Geometry: final body of the model. Coordinates: model frame, mm. A direction names the side the tool comes from. Coordinates: 2 decimals unless noted, no trailing zeros. Write each loop counter-clockwise with the first axis right and the second up, starting at its lowest first coordinate (ties: lowest second). Pieces come first, ordered by that corner, then holes. Notation, with made-up numbers: M 32.5,43 L 63.5,43 A22 cw 63.5,62 Z; hole C 3.5,-10.5 d5. An arc over 180 degrees is marked long. Write item = value, one per line. Start each with the question number.
Item 1: First-contact query: pin 1 Ø5.5 at (y, z) = (28.5, 5.5) entering from +X; pin 2 Ø22.5 at (x, y) = (0, 0) entering from -Z; pin 3 Ø6 at (y, z) = (-35.5, 10) entering from -X; pin 4 Ø8 at (x, z) = (56.5, 16) entering from +Y. Flat tips, straight axial feed; report the tip coordinate or a pass-through.
Item 2: Pull-direction query (Y, two-part tool) for faces 5 (the cylindrical face through (107.144, 43.072, 9.392)), 6 (the cylindrical face through (-107.144, -43.072, 9.392)), 7 (the cylindrical face through (-2.447, 18.636, 9.658)); classes: +Y half, -Y half, draft (parallel to the pull), parting line (faces both ways), or undercut.
Item 3: Reachability of faces 1 (the flat face through (-89.154, -28, 10)), 2 (the flat face through (-19, 50.8, 9)), 3 (the cylindrical face through (18.414, 37.974, 9.658)), 4 (the flat face through (48.006, 28, 10)) from +Z, -Z, +X, -X, +Y, -Y: full face, straight path, thin tool, end or side. Return the list, or none.
Item 4: Section D-D on y = 38.1. Output: boundary loops of the cut face in (x, z) (3 decimals).
Item 5: Section B-B on x = 0. Output: boundary loops of the cut face in (y, z) (3 decimals).
Item 6: Ray query, L1, parallel to Y at x = 0, z = 7.25 (3 decimals); L2, parallel to X at y = 14, z = 12.75; L3, parallel to Y at x = -68, z = 5. Return the intervals inside material, ascending. Write a range as [from, to].
Item 7: Section A-A on z = 7.25. Output: boundary loops of the cut face in (x, y) (1 decimal).
Item 8: Section C-C on y = -15. Output: boundary loops of the cut face in (x, z), plus the area to 3 significant figures.
from build123d import *

# Parameters (mm, degrees)
F1_DEPTH = 19.05
F2_R     = 18.796
F3_DEPTH = 19.051
F5_DEPTH = 19.051
F7_DEPTH = 19.051


with BuildPart() as f1:
    # F0 (on Top) → F1 (new body)
    with BuildSketch(Plane.XY):
        with BuildLine():
            ThreePointArc((114.3, 25.4), (106.860512, 43.360512), (88.9, 50.8))
            Line((88.9, 50.8), (-88.9, 50.8))
            ThreePointArc((-88.9, 50.8), (-106.860512, 43.360512), (-114.3, 25.4))
            Line((-114.3, 25.4), (-114.3, -25.4))
            ThreePointArc((-114.3, -25.4), (-106.860512, -43.360512), (-88.9, -50.8))
            Line((-88.9, -50.8), (88.9, -50.8))
            ThreePointArc((88.9, -50.8), (106.860512, -43.360512), (114.3, -25.4))
            Line((114.3, -25.4), (114.3, 25.4))
        make_face()
    extrude(amount=F1_DEPTH)

    # F2 (on face) → F3 (cut, through all)
    with BuildSketch(Plane.XY.offset(19.05)):
        Circle(F2_R)
    extrude(amount=-F3_DEPTH, mode=Mode.SUBTRACT)

    # F4 (on face) → F5 (cut, through all)
    with BuildSketch(Plane.XY.offset(19.05)):
        with BuildLine():
            Line((-48.006, -50.8), (-48.006, -5.406457))
            ThreePointArc((-48.006, -5.406457), (-68.58, 21.2725), (-89.154, -5.406457))
            Line((-89.154, -5.406457), (-89.154, -50.8))
            Line((-89.154, -50.8), (-48.006, -50.8))
        make_face()
        with BuildLine():
            ThreePointArc((48.006, 5.406457), (68.58, -21.2725), (89.154, 5.406457))
            Line((89.154, 5.406457), (89.154, 50.8))
            Line((89.154, 50.8), (48.006, 50.8))
            Line((48.006, 50.8), (48.006, 5.406457))
        make_face()
    extrude(amount=-F5_DEPTH, mode=Mode.SUBTRACT)

    # F6 (on face) → F7 (cut, through all)
    with BuildSketch(Plane.XY.offset(19.05)):
        with BuildLine():
            ThreePointArc((-12.7, 43.815), (-18.415, 38.1), (-12.7, 32.385))
            Line((-12.7, 32.385), (12.7, 32.385))
            ThreePointArc((12.7, 32.385), (18.415, 38.1), (12.7, 43.815))
            Line((12.7, 43.815), (-12.7, 43.815))
        make_face()
    extrude(amount=-F7_DEPTH, mode=Mode.SUBTRACT)


solid = f1.part
Responses:
q1.pin_1 = 114.3
q1.pin_2 = through
q1.pin_3 = -113.29
q1.pin_4 = -13.93
q2.face_5 = +Y half
q2.face_6 = -Y half
q2.face_7 = undercut
q3.face_1 = +Z, -Z, -Y
q3.face_2 = +Z, -Z, +X, -X, +Y
q3.face_3 = +Z, -Z
q3.face_4 = +Z, -Z, +Y
q4.outline = M -110.897,0 L -18.415,0 L -18.415,19.05 L -110.897,19.05 Z; M 18.415,0 L 48.006,0 L 48.006,19.05 L 18.415,19.05 Z; M 89.154,0 L 110.897,0 L 110.897,19.05 L 89.154,19.05 Z
q5.outline = M -50.8,0 L -18.796,0 L -18.796,19.05 L -50.8,19.05 Z; M 18.796,0 L 32.385,0 L 32.385,19.05 L 18.796,19.05 Z; M 43.815,0 L 50.8,0 L 50.8,19.05 L 43.815,19.05 Z
q6.L1 = [-50.8, -18.796], [18.796, 32.385], [43.815, 50.8]
q6.L2 = [-114.3, -84.6], [-52.56, -12.54], [12.54, 48.01], [89.15, 114.3]
q6.L3 = [21.26, 50.8]
q7.outline = M -114.3,-25.4 A25.4 ccw -89.2,-50.8 L -89.2,-5.4 A21.3 cw long -48,-5.4 L -48,-50.8 L 88.9,-50.8 A25.4 ccw 114.3,-25.4 L 114.3,25.4 A25.4 ccw 89.2,50.8 L 89.2,5.4 A21.3 cw long 48,5.4 L 48,50.8 L -88.9,50.8 A25.4 ccw -114.3,25.4 Z; hole C 0,0 d37.6; hole M -12.7,32.4 L 12.7,32.4 A5.7 ccw 12.7,43.8 L -12.7,43.8 A5.7 ccw Z
q8.outline = M -114.3,0 L -89.15,0 L -89.15,19.05 L -114.3,19.05 Z; M -48.01,0 L -11.33,0 L -11.33,19.05 L -48.01,19.05 Z; M 11.33,0 L 53.5,0 L 53.5,19.05 L 11.33,19.05 Z; M 83.66,0 L 114.3,0 L 114.3,19.05 L 83.66,19.05 Z
q8.area = 2,560 mm²
